```python
from build123d import *

# Parameters (mm, degrees)
F0_W           = 108
F0_H           = 70
F0_W_2         = 105.9
F0_H_2         = 67.9
F0_W_3         = 104
F0_H_3         = 66
F0_R           = 3
F1_DEPTH       = 2
F2_DEPTH       = 10.99
F3_DEPTH       = 10.1
F4_R           = 3.5
F5_DEPTH       = 2
F7_D           = 3.302
F7_CSINK_D     = 6.477
F7_CSINK_ANGLE = 82
F8_W           = 21
F8_H           = 6.4
F9_DEPTH       = 2.5
F10_W          = 13
F10_H          = 0.95
F11_DEPTH      = 2.5
F13_DEPTH      = 2.5
F14_R          = 1.5
F15_R          = 1.5
F16_W          = 21
F16_H          = 0.89
F17_DEPTH      = 2.5


# Not quite as in the source:
# - a feature names something its author has since deleted; it is built from what else it names


with BuildPart() as f1:
    # F0 (on Top) → F1 (new body)
    with BuildSketch(Plane.XY):
        with Locations((9.6408709802, -2.0854342729)):
            Rectangle(F0_W, F0_H)
        with Locations((9.6408709802, -2.0854342729)):
            Rectangle(F0_W_2, F0_H_2, mode=Mode.SUBTRACT)
        with Locations((9.6408709802, -2.0854342729)):
            Rectangle(F0_W_2, F0_H_2)
        with Locations((9.6408709802, -2.0854342729)):
            Rectangle(F0_W_3, F0_H_3, mode=Mode.SUBTRACT)
        with Locations((9.6408709802, -2.0854342729)):
            Rectangle(F0_W_3, F0_H_3)
        with Locations((-36.8591290198, -29.5854342729)):
            Circle(F0_R, mode=Mode.SUBTRACT)
        with Locations((54.9200624228, -29.5854342729)):
            Circle(F0_R, mode=Mode.SUBTRACT)
        with Locations((-36.8591290198, 25.4145657271)):
            Circle(F0_R, mode=Mode.SUBTRACT)
        with Locations((57.1408709802, 25.4145657271)):
            Circle(F0_R, mode=Mode.SUBTRACT)
        with Locations((-36.8591290198, -29.5854342729)):
            Circle(F0_R)
        with Locations((54.9200624228, -29.5854342729)):
            Circle(F0_R)
        with Locations((-36.8591290198, 25.4145657271)):
            Circle(F0_R)
        with Locations((57.1408709802, 25.4145657271)):
            Circle(F0_R)
    extrude(amount=-F1_DEPTH)

    # F0 (on Top) → F2 (join)
    with BuildSketch(Plane.XY):
        with Locations((9.6408709802, -2.0854342729)):
            Rectangle(F0_W_2, F0_H_2)
        with Locations((9.6408709802, -2.0854342729)):
            Rectangle(F0_W_3, F0_H_3, mode=Mode.SUBTRACT)
    extrude(amount=F2_DEPTH)

    # F0 (on Top) → F3 (join)
    with BuildSketch(Plane.XY):
        with Locations((9.6408709802, -2.0854342729)):
            Rectangle(F0_W, F0_H)
        with Locations((9.6408709802, -2.0854342729)):
            Rectangle(F0_W_2, F0_H_2, mode=Mode.SUBTRACT)
    extrude(amount=F3_DEPTH)

    # F4 (on face) → F5 (join)
    with BuildSketch(Plane.XY):
        with Locations((-36.8591290198, 25.4145657271)):
            Circle(F4_R)
        with Locations((56.1408709802, 25.4145657271)):
            Circle(F4_R)
        with Locations((56.1408709802, -29.5854342729)):
            Circle(F4_R)
        with Locations((-36.8591290198, -29.5854342729)):
            Circle(F4_R)
    extrude(amount=F5_DEPTH)

    # F7 (through all)
    with Locations(Plane(origin=(0, 0, -2), x_dir=(1, 0, 0), z_dir=(0, 0, -1))):
        with Locations((-36.8591290198, 29.5854342729), (56.1408709802, 29.5854342729), (56.1408709802, -25.4145657271), (-36.8591290198, -25.4145657271)):
            CounterSinkHole(F7_D / 2, F7_CSINK_D / 2, counter_sink_angle=F7_CSINK_ANGLE)

    # F8 (on face) → F9 (cut)
    with BuildSketch(Plane(origin=(0, 32.9145657271, 0), x_dir=(-1, 0, 0), z_dir=(0, 1, 0))):
        with Locations((-31.5408709802, 6.9)):
            Rectangle(F8_W, F8_H)
    extrude(amount=-F9_DEPTH, mode=Mode.SUBTRACT)

    # F10 (on face) → F11 (cut)
    with BuildSketch(Plane.XY.offset(10.99)):
        with Locations((38.6408709802, -35.5604342729)):
            Rectangle(F10_W, F10_H)
    extrude(amount=-F11_DEPTH, mode=Mode.SUBTRACT)

    # F12 (on face) → F13 (cut)
    with BuildSketch(Plane.XZ.offset(37.0854342729)):
        with BuildLine():
            ThreePointArc((32.1408709802, 10.1), (38.6408709802, 3.6), (45.1408709802, 10.1))
            Line((45.1408709802, 10.1), (32.1408709802, 10.1))
        make_face()
    extrude(amount=-F13_DEPTH, mode=Mode.SUBTRACT)

    # F14
    f14_edges = [f1.edges().sort_by_distance(p)[0] for p in [
        (63.640871, -37.085434, 4.05),
        (63.640871, -2.085434, -2),
        (63.640871, 32.914566, 4.05),
        (9.640871, 32.914566, -2),
        (-44.359129, 32.914566, 4.05),
        (-44.359129, -37.085434, 4.05),
        (-44.359129, -2.085434, -2),
        (9.640871, -37.085434, -2),
    ]]
    fillet(f14_edges, radius=F14_R)

    # F15
    f15_edges = [f1.edges().sort_by_distance(p)[0] for p in [
        (9.640871, 30.914566, 0),
        (-42.359129, 30.914566, 5.495),
        (-42.359129, -2.085434, 0),
        (9.640871, -35.085434, 0),
        (-42.359129, -35.085434, 5.495),
        (61.640871, 30.914566, 5.495),
        (61.640871, -2.085434, 0),
        (61.640871, -35.085434, 5.495),
    ]]
    fillet(f15_edges, radius=F15_R)

    # F16 (on face) → F17 (cut)
    with BuildSketch(Plane(origin=(0, 31.8645657271, 0), x_dir=(-1, 0, 0), z_dir=(0, 1, 0))):
        with Locations((-31.5408709802, 10.545)):
            Rectangle(F16_W, F16_H)
    extrude(amount=-F17_DEPTH, mode=Mode.SUBTRACT)


solid = f1.part
```
Here's how the part is built. I have some questions about the finished solid (model axes, mm). A direction names the side the tool comes from. Coordinates: 2 decimals unless noted, no trailing zeros. Order: outer loops, then holes, each group sorted by start corner. A loop starts at its lowest first (then second) coordinate and runs counter-clockwise, first axis right, second up. Notation, with made-up numbers: (13.5, 3) -> (71.5, 3) arc R20 ccw to (71.5, 18) -> close; hole circle Ø6 at (-19, 86.25). An arc over 180 degrees is marked (long way). Return JSON: item names as keys, results as strings.
1) If we section it at B-B on y = -10.5: List the corners of the cut face in (x, z) for me, plus the area to 3 significant figures.
Conclusion:
{"outline": "(-44.36, -0.5) arc R1.5 ccw to (-42.86, -2) -> (62.14, -2) arc R1.5 ccw to (63.64, -0.5) -> (63.64, 10.1) -> (62.59, 10.1) -> (62.59, 10.99) -> (61.64, 10.99) -> (61.64, 1.5) arc R1.5 cw to (60.14, 0) -> (-40.86, 0) arc R1.5 cw to (-42.36, 1.5) -> (-42.36, 10.99) -> (-43.31, 10.99) -> (-43.31, 10.1) -> (-44.36, 10.1) -> close", "area": "258 mm²"}
2) On a 3-axis mill with a long thin cutter (end or side, diameter ignored), from which of +Z, -Z, +X, -X, +Y, -Y can I reach the whole of each face in a straight line? I mean faces 1 (the flat face through (62, -2, 10.99)), 2 (the cylindrical face through (-37.747, -30.978, 0.928)), 3 (the cylindrical face through (38.5, -36.1, 3.6)), 4 (the flat face through (21.041, 32, 7)), 5 (the flat face through (9, 30.915, 6)). Say none if no direction works.
Conclusion:
{"face 1": "+Z, +X, -X, +Y, -Y", "face 2": "+Z, -Z", "face 3": "+Z, -Y", "face 4": "+Z, +Y", "face 5": "+Z"}
3) I'm going to push flat-ended pins straight in: P1, Ø5.5, axis at x = 56.5, y = -30, coming from the +Z side; P2, Ø1, axis at x = 26.5, y = -18.5, coming from the +Z side; P3, Ø2, axis at x = 56.14, y = -29.59, coming from the -Z side. Where does each tip first touch, or does it pass through?
Conclusion:
{"P1": "stops at z = 2", "P2": "stops at z = 0", "P3": "passes through"}
4) If we section it at A-A on x = 28: List the corners of the cut face in (y, z) for me.
Conclusion:
{"outline": "(-37.09, -0.5) arc R1.5 ccw to (-35.59, -2) -> (31.41, -2) arc R1.5 ccw to (32.91, -0.5) -> (32.91, 3.7) -> (30.91, 3.7) -> (30.91, 1.5) arc R1.5 cw to (29.41, 0) -> (-33.59, 0) arc R1.5 cw to (-35.09, 1.5) -> (-35.09, 10.99) -> (-36.04, 10.99) -> (-36.04, 10.1) -> (-37.09, 10.1) -> close"}
5) If I drill on probe 1 along Y at (x, z) = (52, 5.75); probe 2 along X at (y, z) = (-20, 1.25); probe 3 along X at (y, z) = (-30, 6.5), over which ranges is the centre line in solid material (lowest first)?
Conclusion:
{"probe 1": "y = -37.09 to -35.09, 30.91 to 32.91", "probe 2": "x = -44.36 to -42.34, 61.62 to 63.64", "probe 3": "x = -44.36 to -42.36, 61.64 to 63.64"}
6) Thinking about a two-plate mould opening in Y: for faces 6 (the cylindrical face through (57.36, -30.7, 0.93)), 7 (the flat face through (63.641, -3, 5)), 8 (the flat face through (9, 32.915, 5)), which applies, +Y half, -Y half, draft (parallel to the pull), parting line (faces both ways), or undercut?
Conclusion:
{"face 6": "undercut", "face 7": "draft", "face 8": "+Y half"}
